Read the model definition and answer for the solid it produces. Units are mm, in the model's axes. Face numbers are marked on the shaded views. A direction names the side the tool comes from. Round coordinates to 2 decimals unless told otherwise and drop trailing zeros. Write each loop counter-clockwise with the first axis right and the second up, starting at its lowest first coordinate (ties: lowest second). Pieces come first, ordered by that corner, then holes. Notation, with made-up numbers: (24.5, 0.5) - (42.5, 0.5) arc R28 cw to (42.5, 23.5) - close; hole circle Ø11 at (31, -14). An arc over 180 degrees is marked (long way). One line per item, written item: value. Start each with the question number.
(1) Flat-ended cylindrical pins translate along their axes: pin 1 Ø3.5 at (y, z) = (36, 0) entering from -X; pin 2 Ø8 at (x, y) = (7, -28.5) entering from -Z; pin 3 Ø2 at (y, z) = (36.5, 13) entering from +X; pin 4 Ø5 at (x, z) = (13, 16) entering from +Y. Find the tip coordinate at first contact, or state that the pin passes through.
(2) A cutting plane is placed at A-A, the plane z = 0. Determine the outline of the cut face in (x, y).
(3) A cutting plane is placed at B-B, the plane x = 0. Determine the outline of the cut face in (y, z).
(4) For the marked faces 1 and 2, determine the directions among +Z, -Z, +X, -X, +Y, -Y from which every point of the face is accessible in a straight line to the end or side of a thin tool.
(5) A cutting plane is placed at C-C, the plane y = 19.5. Determine the outline of the cut face in (x, z).
(6) Find the intervals of material crossed by L1, parallel to Y at x = 14, z = 11; L2, parallel to Z at x = 0, y = 36; L3, parallel to Z at x = -4.5, y = 36, in increasing order.
(7) A cutting plane is placed at D-D, the plane y = 36. Determine the outline of the cut face in (x, z).
from build123d import *

# Parameters (mm, degrees)
F0_R     = 15
F1_DEPTH = 51
F2_R     = 22.5
F3_DEPTH = 15
F4_R     = 3
F5_DEPTH = 15


with BuildPart() as f1:
    # F0 (on Front) → F1 (new body, symmetric)
    with BuildSketch(Plane.XZ):
        Circle(F0_R)
    extrude(amount=F1_DEPTH, both=True)

    # F2 (on face) → F3 (join)
    with BuildSketch(Plane.XZ.offset(51)):
        Circle(F2_R)
    extrude(amount=F3_DEPTH)

    # F4 (on Right) → F5 (cut, symmetric)
    with BuildSketch(Plane.YZ):
        with Locations((36, 0)):
            Circle(F4_R)
    extrude(amount=F5_DEPTH, both=True, mode=Mode.SUBTRACT)


solid = f1.part
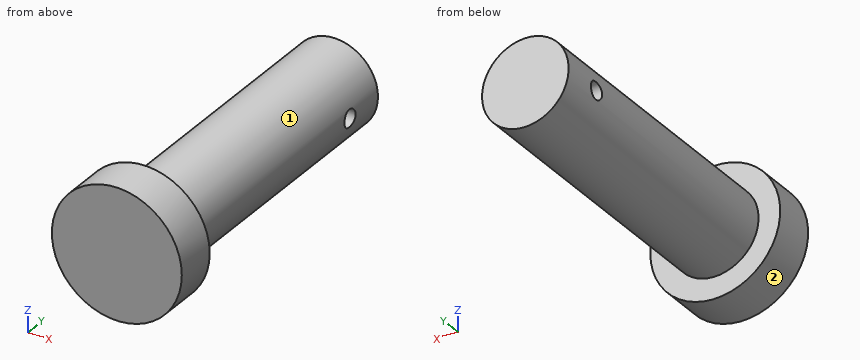
Here are the results:
1. pin 1: through
1. pin 2: z = -14.7
1. pin 3: x = 9
1. pin 4: y = -51
2. outline: (-22.5, -66) - (22.5, -66) - (22.5, -51) - (15, -51) - (15, 33) - (-15, 33) - (-15, -51) - (-22.5, -51) - close; (-15, 39) - (15, 39) - (15, 51) - (-15, 51) - close
3. outline: (-66, -22.5) - (-51, -22.5) - (-51, -15) - (51, -15) - (51, 15) - (-51, 15) - (-51, 22.5) - (-66, 22.5) - close; hole circle Ø6 at (36, 0)
4. face 1: +Y
4. face 2: +Y, -Y
5. outline: circle Ø30 at (0, 0)
6. L1: -66 to -51
6. L2: -15 to -3, 3 to 15
6. L3: -14.31 to -3, 3 to 14.31
7. outline: (-14.7, -3) arc R15 ccw to (14.7, -3) - close; (-14.7, 3) - (14.7, 3) arc R15 ccw to start
